Could you check a few things on this model? Use its own coordinates, in mm. Round coordinates to 2 decimals unless told otherwise and drop trailing zeros. Loops run counter-clockwise (first coordinate to the right, second up) from the corner with the lowest first, then second, coordinate; pieces in that order, holes last. Notation, with made-up numbers: (87, 63) -> (144, 63) arc R11 ccw to (144, 73) -> close; hole circle Ø11 at (-3.75, 45.25). An arc over 180 degrees is marked (long way). One line per item, written item: value.
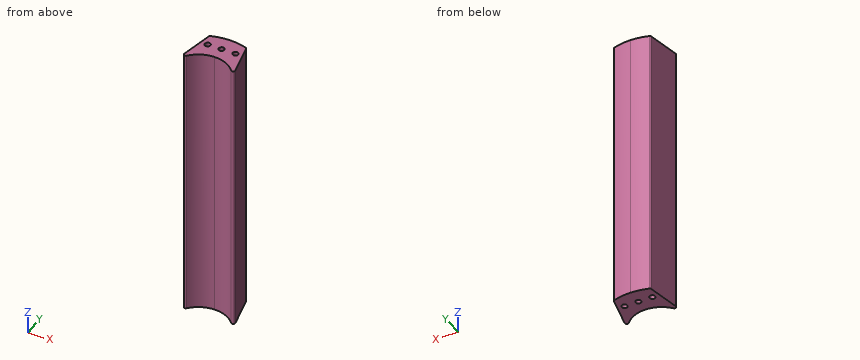
from build123d import *

# Parameters (mm, degrees)
F0_R     = 1.5
F1_DEPTH = 150


with BuildPart() as f1:
    # F0 (on Top) → F1 (new body)
    with BuildSketch(Plane.XY):
        with BuildLine():
            ThreePointArc((0, 16), (6.612297, 14.569747), (12.042437, 10.534691))
            ThreePointArc((12.042437, 10.534691), (13.241723, 10.298392), (13.773683, 11.398912))
            Line((13.773683, 11.398912), (10.118439, 28.779623))
            ThreePointArc((10.118439, 28.779623), (9.88218, 29.24385), (9.444507, 29.526281))
            ThreePointArc((9.444507, 29.526281), (4.779397, 30.629355), (0, 31))
            Line((0, 31), (0, 24.5))
            ThreePointArc((0, 24.5), (1.06066, 24.06066), (1.5, 23))
            ThreePointArc((1.5, 23), (1.06066, 21.93934), (0, 21.5))
            Line((0, 21.5), (0, 16))
        make_face()
        with Locations((7.5, 23)):
            Circle(F0_R, mode=Mode.SUBTRACT)
        with BuildLine():
            ThreePointArc((-12.042437, 10.534691), (-6.612297, 14.569747), (0, 16))
            Line((0, 16), (0, 21.5))
            ThreePointArc((0, 21.5), (-1.5, 23), (0, 24.5))
            Line((0, 24.5), (0, 31))
            ThreePointArc((0, 31), (-4.779397, 30.629355), (-9.444507, 29.526281))
            ThreePointArc((-9.444507, 29.526281), (-9.88218, 29.24385), (-10.118439, 28.779623))
            Line((-10.118439, 28.779623), (-13.773683, 11.398912))
            ThreePointArc((-13.773683, 11.398912), (-13.241723, 10.298392), (-12.042437, 10.534691))
        make_face()
        with Locations((-7.5, 23)):
            Circle(F0_R, mode=Mode.SUBTRACT)
    extrude(amount=F1_DEPTH)


solid = f1.part
(1) I'm going to push flat-ended pins straight in: pin 1 Ø2 at (y, z) = (22.5, 91.5) entering from +X; pin 2 Ø4 at (y, z) = (17, 74) entering from +X; pin 3 Ø1.5 at (x, z) = (-4, 18.5) entering from +Y; pin 4 Ø1.8 at (x, y) = (7.5, 23) entering from -Z. Where does each tip first touch, or does it pass through?
Recorded:
pin 1: x = 11.65
pin 2: x = 13.02
pin 3: y = 30.83
pin 4: through
(2) If we section it at A-A, the plane z = 98: Please give me the cut outline in (x, y), then the cut area to 3 significant figures.
Recorded:
outline: (-13.77, 11.4) arc R1 ccw to (-12.04, 10.53) arc R16 cw to (12.04, 10.53) arc R1 ccw to (13.77, 11.4) -> (10.12, 28.78) arc R1 ccw to (9.44, 29.53) arc R31 ccw to (0, 31) arc R31 ccw to (-9.44, 29.53) arc R1 ccw to (-10.12, 28.78) -> close; hole circle Ø3 at (-7.5, 23); hole circle Ø3 at (0, 23); hole circle Ø3 at (7.5, 23)
area: 361 mm²
(3) If we section it at B-B, the plane x = -7.5: Please give me the cut outline in (y, z).
Recorded:
outline: (14.13, 0) -> (21.5, 0) -> (21.5, 150) -> (14.13, 150) -> close; (24.5, 0) -> (30.08, 0) -> (30.08, 150) -> (24.5, 150) -> close
(4) If we section it at C-C, the plane y = 20: Please give me the cut outline in (x, z), then the cut area to 3 significant figures.
Recorded:
outline: (-11.96, 0) -> (11.96, 0) -> (11.96, 150) -> (-11.96, 150) -> close
area: 3,590 mm²
(5) If I drill on L1, parallel to X at y = 22, z = 52; L2, parallel to Y at x = -6.5, z = 102; L3, parallel to Y at x = -7.5, z = 102, over which ranges is the centre line in solid material (lowest first)?
Recorded:
L1: -11.54 to -8.62, -6.38 to -1.12, 1.12 to 6.38, 8.62 to 11.54
L2: 14.62 to 21.88, 24.12 to 30.31
L3: 14.13 to 21.5, 24.5 to 30.08
